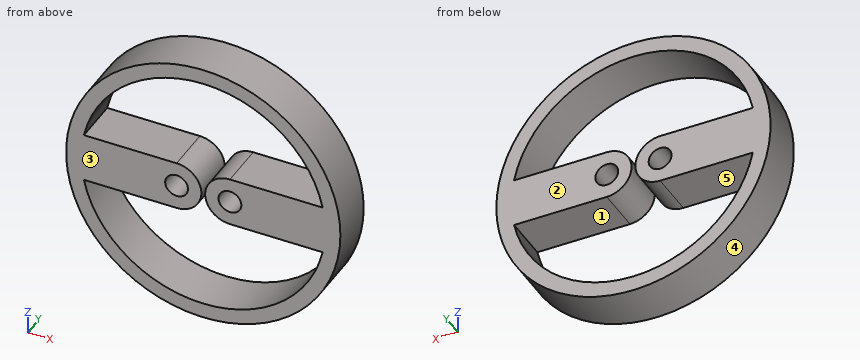
from build123d import *

# Parameters (mm, degrees)
ESQUISSE1_R        = 18
ESQUISSE1_R_2      = 1.5
BOSS_EXTRU_1_DEPTH = 6


with BuildPart() as part:
    # Esquisse1 → Boss.-Extru.1 (new body)
    with BuildSketch(Plane(origin=(0, 0, 0), x_dir=(1, 0, 0), z_dir=(0, 1, 0))):
        Circle(ESQUISSE1_R)
        with Locations((-3.5, 0)):
            Circle(ESQUISSE1_R_2, mode=Mode.SUBTRACT)
        with Locations((3.5, 0)):
            Circle(ESQUISSE1_R_2, mode=Mode.SUBTRACT)
        with BuildLine():
            Line((-3.5, 3.25), (-15.666445034, 3.25))
            ThreePointArc((-15.666445034, 3.25), (0, 16), (15.666445034, 3.25))
            Line((15.666445034, 3.25), (3.5, 3.25))
            ThreePointArc((3.5, 3.25), (0.25, 0), (3.5, -3.25))
            Line((3.5, -3.25), (15.666445034, -3.25))
            ThreePointArc((15.666445034, -3.25), (0, -16), (-15.666445034, -3.25))
            Line((-15.666445034, -3.25), (-3.5, -3.25))
            ThreePointArc((-3.5, -3.25), (-0.25, 0), (-3.5, 3.25))
        make_face(mode=Mode.SUBTRACT)
    extrude(amount=BOSS_EXTRU_1_DEPTH)


solid = part.part
Here's how the part is built. I have some questions about the finished solid (model axes, mm). Face numbers are marked on the shaded views. A direction names the side the tool comes from. Coordinates: 2 decimals unless noted, no trailing zeros. Order: outer loops, then holes, each group sorted by start corner. A loop starts at its lowest first (then second) coordinate and runs counter-clockwise, first axis right, second up. Notation, with made-up numbers: (-3, 76) - (39, 76) arc R9 cw to (39, 84) - close; hole circle Ø2 at (83.25, 1). An arc over 180 degrees is marked (long way). Use CSV: the item, a comma, the result in double quotes. Start each with the question number.
1. Suppose I cut it at D-D on x = -8.5. List the corners of the cut face in (y, z) for me, then the cut area to 3 significant figures.
2. Suppose I cut it at C-C on x = -4.5. List the corners of the cut face in (y, z) for me.
3. Suppose I cut it at B-B on y = 3.9. List the corners of the cut face in (x, z) for me.
4. Suppose I cut it at A-A on z = 0. List the corners of the cut face in (x, y) for me.
5. I'm going to push flat-ended pins straight in: pin 1 (1.5 mm diameter, centred on y = 4, z = 8, fed in from +X); pin 2 (1 mm diameter, centred on x = 4, y = 2.5, fed in from -Z); pin 3 (1.8 mm diameter, centred on x = -11, y = 3, fed in from +Z). Where does each tip first touch, or does it pass through?
6. Please list where these lines run through material, in increasing order: line 1 (X direction, y = 2.7, z = 0); line 2 (Z direction, x = -4.5, y = 5.05); line 3 (Z direction, x = -9, y = 4.2). Write a range as from..to.
7. If we mould it in two halves opening along X, with no side actions, what happens to the marked faces 3, 4 and 5? For each: +X half, -X half, draft (parallel to the pull), parting line (faces both ways), or undercut.
8. For the marked faces 1 and 2, which set-ups out of +Z, -Z, +X, -X, +Y, -Y let a thin tool reach every point of the face, with its end or its side?
Output:
1,outline,"(0, -15.87) - (6, -15.87) - (6, -13.56) - (0, -13.56) - close; (0, -3.25) - (6, -3.25) - (6, 3.25) - (0, 3.25) - close; (0, 13.56) - (6, 13.56) - (6, 15.87) - (0, 15.87) - close"
1,area,"66.7 mm2"
2,outline,"(0, -17.43) - (6, -17.43) - (6, -15.35) - (0, -15.35) - close; (0, -3.25) - (6, -3.25) - (6, -1.12) - (0, -1.12) - close; (0, 1.12) - (6, 1.12) - (6, 3.25) - (0, 3.25) - close; (0, 15.35) - (6, 15.35) - (6, 17.43) - (0, 17.43) - close"
3,outline,"circle Ø36 at (0, 0); hole (-15.67, -3.25) arc R16 ccw to (15.67, -3.25) - (3.5, -3.25) arc R3.25 cw to (3.5, 3.25) - (15.67, 3.25) arc R16 ccw to (-15.67, 3.25) - (-3.5, 3.25) arc R3.25 cw to (-3.5, -3.25) - close; hole circle Ø3 at (-3.5, 0); hole circle Ø3 at (3.5, 0)"
4,outline,"(-18, 0) - (-5, 0) - (-5, 6) - (-18, 6) - close; (-2, 0) - (-0.25, 0) - (-0.25, 6) - (-2, 6) - close; (0.25, 0) - (2, 0) - (2, 6) - (0.25, 6) - close; (5, 0) - (18, 0) - (18, 6) - (5, 6) - close"
5,pin 1,"stops at x = 16.48"
5,pin 2,"stops at z = -17.66"
5,pin 3,"stops at z = 14.9"
6,line 1,"x = -18..-5, -2..-0.25, 0.25..2, 5..18"
6,line 2,"z = -17.43..-15.35, -3.25..-1.12, 1.12..3.25, 15.35..17.43"
6,line 3,"z = -15.59..-13.23, -3.25..3.25, 13.23..15.59"
7,face 3,"draft"
7,face 4,"parting line"
7,face 5,"undercut"
8,face 1,"+Y, -Y"
8,face 2,"+Z, -Z, +X, -X, +Y"
